The listing builds one solid part. Answer for the finished solid, in the listing's coordinates (mm). Face numbers are marked on the shaded views. A direction names the side the tool comes from. Round coordinates to 2 decimals unless told otherwise and drop trailing zeros. One line per item, written item: value.
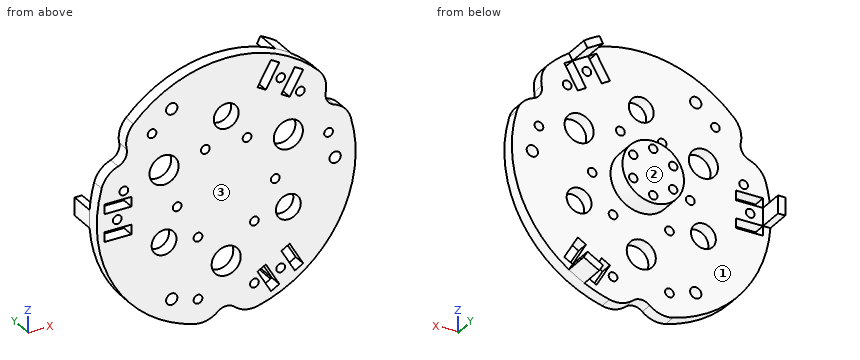
```python
from build123d import *

# Parameters (mm, degrees)
SKETCH1_R                = 50.5
BOSS_EXTRUDE1_DEPTH      = 5
SKETCH3_R                = 12
SKETCH3_R_2              = 1.65
BOSS_EXTRUDE2_DEPTH      = 8
CUT_EXTRUDE6_REACH       = 73.864
SKETCH9_R                = 5.675
SKETCH9_R_2              = 1.7
CIRPATTERN1_COUNT        = 3
SKETCH10_R               = 4.85
CUT_EXTRUDE7_DEPTH       = 72.864455748
SKETCH11_R               = 1.7
CUT_EXTRUDE8_DEPTH       = 72.864455748
CUT_EXTRUDE9_REACH       = 73.864
SKETCH13_R               = 2.2
CIRPATTERN2_COUNT        = 3
CUT_EXTRUDE11_DEPTH      = 72.864455748
BOSS_EXTRUDE3_DEPTH      = 10
CIRPATTERN3_COUNT        = 3
CUT_EXTRUDE12_DEPTH      = 73.114492302
FILLET1_R                = 10
CIRPATTERN4_COUNT        = 3
FILLET1_OF_CIRPATTERN4_R = 10


with BuildPart() as part:
    # Sketch1 → Boss-Extrude1 (new body)
    with BuildSketch(Plane(origin=(0, 0, 0), x_dir=(1, 0, 0), z_dir=(0, 1, 0))):
        with Locations(Location((0, 0, 0), (0, 0, 270))):
            Circle(SKETCH1_R)
    extrude(amount=BOSS_EXTRUDE1_DEPTH)

    # Sketch3 → Boss-Extrude2 (add)
    with BuildSketch(Plane(origin=(0, 5, 0), x_dir=(1, 0, 0), z_dir=(0, 1, 0))):
        with Locations(Location((0, 0, 0), (0, 0, 270))):
            Circle(SKETCH3_R)
        with Locations(Location((0, 9, 0), (0, 0, 270))):
            Circle(SKETCH3_R_2, mode=Mode.SUBTRACT)
        with Locations(Location((7.794228634, 4.5, 0), (0, 0, 270))):
            Circle(SKETCH3_R_2, mode=Mode.SUBTRACT)
        with Locations(Location((7.794228634, -4.5, 0), (0, 0, 270))):
            Circle(SKETCH3_R_2, mode=Mode.SUBTRACT)
        with Locations(Location((0, -9, 0), (0, 0, 270))):
            Circle(SKETCH3_R_2, mode=Mode.SUBTRACT)
        with Locations(Location((-7.794228634, -4.5, 0), (0, 0, 270))):
            Circle(SKETCH3_R_2, mode=Mode.SUBTRACT)
        with Locations(Location((-7.794228634, 4.5, 0), (0, 0, 270))):
            Circle(SKETCH3_R_2, mode=Mode.SUBTRACT)
    extrude(amount=BOSS_EXTRUDE2_DEPTH)

    # Sketch9 → Cut-Extrude6 (cut, up to next)
    with BuildSketch(Plane(origin=(0, 5, 0), x_dir=(1, 0, 0), z_dir=(0, 1, 0)), mode=Mode.PRIVATE) as cut_extrude6_sk1:
        with Locations(Location((0, 28, 0), (0, 0, 270))):
            Circle(SKETCH9_R)
    cut_extrude6_tool1 = extrude(cut_extrude6_sk1.sketch, amount=-CUT_EXTRUDE6_REACH, mode=Mode.PRIVATE) & part.part
    # Sketch9 → Cut-Extrude6 (cut, up to next)
    with BuildSketch(Plane(origin=(0, 5, 0), x_dir=(1, 0, 0), z_dir=(0, 1, 0)), mode=Mode.PRIVATE) as cut_extrude6_sk2:
        with Locations(Location((11, 15.75, 0), (0, 0, 270))):
            Circle(SKETCH9_R_2)
    cut_extrude6_tool2 = extrude(cut_extrude6_sk2.sketch, amount=-CUT_EXTRUDE6_REACH, mode=Mode.PRIVATE) & part.part
    # Sketch9 → Cut-Extrude6 (cut, up to next)
    with BuildSketch(Plane(origin=(0, 5, 0), x_dir=(1, 0, 0), z_dir=(0, 1, 0)), mode=Mode.PRIVATE) as cut_extrude6_sk3:
        with Locations(Location((-11, 15.75, 0), (0, 0, 270))):
            Circle(SKETCH9_R_2)
    cut_extrude6_tool3 = extrude(cut_extrude6_sk3.sketch, amount=-CUT_EXTRUDE6_REACH, mode=Mode.PRIVATE) & part.part
    # Sketch9 → Cut-Extrude6 (cut, up to next)
    with BuildSketch(Plane(origin=(0, 5, 0), x_dir=(1, 0, 0), z_dir=(0, 1, 0)), mode=Mode.PRIVATE) as cut_extrude6_sk4:
        with Locations(Location((11, 39.75, 0), (0, 0, 270))):
            Circle(SKETCH9_R_2)
    cut_extrude6_tool4 = extrude(cut_extrude6_sk4.sketch, amount=-CUT_EXTRUDE6_REACH, mode=Mode.PRIVATE) & part.part
    # Sketch9 → Cut-Extrude6 (cut, up to next)
    with BuildSketch(Plane(origin=(0, 5, 0), x_dir=(1, 0, 0), z_dir=(0, 1, 0)), mode=Mode.PRIVATE) as cut_extrude6_sk5:
        with Locations(Location((-11, 39.75, 0), (0, 0, 270))):
            Circle(SKETCH9_R_2)
    cut_extrude6_tool5 = extrude(cut_extrude6_sk5.sketch, amount=-CUT_EXTRUDE6_REACH, mode=Mode.PRIVATE) & part.part
    cut_extrude6_1 = cut_extrude6_tool1.solids().sort_by_distance((0, 5, -28))[0]
    add(cut_extrude6_1, mode=Mode.SUBTRACT)
    cut_extrude6_2 = cut_extrude6_tool2.solids().sort_by_distance((11, 5, -15.75))[0]
    add(cut_extrude6_2, mode=Mode.SUBTRACT)
    cut_extrude6_3 = cut_extrude6_tool3.solids().sort_by_distance((-11, 5, -15.75))[0]
    add(cut_extrude6_3, mode=Mode.SUBTRACT)
    cut_extrude6_4 = cut_extrude6_tool4.solids().sort_by_distance((11, 5, -39.75))[0]
    add(cut_extrude6_4, mode=Mode.SUBTRACT)
    cut_extrude6_5 = cut_extrude6_tool5.solids().sort_by_distance((-11, 5, -39.75))[0]
    add(cut_extrude6_5, mode=Mode.SUBTRACT)
    cut_extrude6 = cut_extrude6_1 + cut_extrude6_2 + cut_extrude6_3 + cut_extrude6_4 + cut_extrude6_5  # Cut-Extrude6 as one shape, for the pattern or mirror that repeats it

    # CirPattern1: Cut-Extrude6 ×3 about axis
    cirpattern1_axis = Axis((0, 0, 0), (0, 1, 0))
    for i in range(1, CIRPATTERN1_COUNT):
        add(cut_extrude6.rotate(cirpattern1_axis, i * 360 / CIRPATTERN1_COUNT), mode=Mode.SUBTRACT)

    # Sketch10 → Cut-Extrude7 (cut, through all)
    with BuildSketch(Plane(origin=(0, 5, 0), x_dir=(1, 0, 0), z_dir=(0, 1, 0))):
        with Locations(Location((-24.248711306, 14, 0), (0, 0, 270))):
            Circle(SKETCH10_R)
        with Locations(Location((24.248711306, 14, 0), (0, 0, 270))):
            Circle(SKETCH10_R)
        with Locations(Location((0, -28, 0), (0, 0, 270))):
            Circle(SKETCH10_R)
    extrude(amount=-CUT_EXTRUDE7_DEPTH, mode=Mode.SUBTRACT)

    # Sketch11 → Cut-Extrude8 (cut, through all)
    with BuildSketch(Plane(origin=(0, 5, 0), x_dir=(1, 0, 0), z_dir=(0, 1, 0))):
        with Locations(Location((21.25, 36.806079661, 0), (0, 0, 270))):
            Circle(SKETCH11_R)
    cut_extrude8 = extrude(amount=-CUT_EXTRUDE8_DEPTH, mode=Mode.SUBTRACT)

    # Sketch13 → Cut-Extrude9 (cut, up to next)
    with BuildSketch(Plane(origin=(0, 5, 0), x_dir=(1, 0, 0), z_dir=(0, 1, 0)), mode=Mode.PRIVATE) as cut_extrude9_sk1:
        with Locations(Location((-21.25, 36.806079661, 0), (0, 0, 270))):
            Circle(SKETCH13_R)
    cut_extrude9_tool1 = extrude(cut_extrude9_sk1.sketch, amount=-CUT_EXTRUDE9_REACH, mode=Mode.PRIVATE) & part.part
    cut_extrude9 = cut_extrude9_tool1.solids().sort_by_distance((-21.25, 5, -36.80608))[0]
    add(cut_extrude9, mode=Mode.SUBTRACT)

    # CirPattern2: Cut-Extrude8, Cut-Extrude9 ×3 about axis
    cirpattern2_axis = Axis((0, 0, 0), (0, 1, 0))
    add([cut_extrude8.rotate(cirpattern2_axis, i * 360 / CIRPATTERN2_COUNT) for i in range(1, CIRPATTERN2_COUNT)], mode=Mode.SUBTRACT)
    add([cut_extrude9.rotate(cirpattern2_axis, i * 360 / CIRPATTERN2_COUNT) for i in range(1, CIRPATTERN2_COUNT)], mode=Mode.SUBTRACT)

    # Sketch15 → Cut-Extrude11 (cut, through all)
    with BuildSketch(Plane(origin=(0, 5, 0), x_dir=(1, 0, 0), z_dir=(0, 1, 0))):
        Polygon((20.718911087, 42.88620668), (17.471315823, 44.76120668), (12.221315823, 35.66793994), (15.468911087, 33.79293994), align=None)
        Polygon((26.781088913, 39.38620668), (30.028684177, 37.51120668), (24.778684177, 28.41793994), (21.531088913, 30.29293994), align=None)
    cut_extrude11 = extrude(amount=-CUT_EXTRUDE11_DEPTH, mode=Mode.SUBTRACT)

    # Sketch17 → Boss-Extrude3 (add)
    with BuildSketch(Plane(origin=(0, 5, 0), x_dir=(1, 0, 0), z_dir=(0, 1, 0))):
        with BuildLine():
            Line((20.718911087, 42.88620668), (26.781088913, 39.38620668))
            Line((26.781088913, 39.38620668), (28.220372349, 41.879118717))
            ThreePointArc((28.220372349, 41.879118717), (25.25, 43.734282891), (22.158194522, 45.379118717))
            Line((22.158194522, 45.379118717), (20.718911087, 42.88620668))
        make_face()
    boss_extrude3 = extrude(amount=BOSS_EXTRUDE3_DEPTH)

    # CirPattern3: Cut-Extrude11, Boss-Extrude3 ×3 about axis
    cirpattern3_axis = Axis((0, 0, 0), (0, 1, 0))
    add([cut_extrude11.rotate(cirpattern3_axis, i * 360 / CIRPATTERN3_COUNT) for i in range(1, CIRPATTERN3_COUNT)], mode=Mode.SUBTRACT)
    add([boss_extrude3.rotate(cirpattern3_axis, i * 360 / CIRPATTERN3_COUNT) for i in range(1, CIRPATTERN3_COUNT)])

    # Sketch18 → Cut-Extrude12 (cut, through all)
    with BuildSketch(Plane(origin=(0, 5, 0), x_dir=(1, 0, 0), z_dir=(0, 1, 0))):
        with BuildLine():
            ThreePointArc((41.022985472, -29.45105538), (43.734282891, -25.25), (46.016854863, -20.801419868))
            ThreePointArc((46.016854863, -20.801419868), (39.404155872, -22.75), (41.022985472, -29.45105538))
        make_face()
    cut_extrude12 = extrude(amount=-CUT_EXTRUDE12_DEPTH, mode=Mode.SUBTRACT)

    # Fillet1
    fillet1_edges = [part.edges().sort_by_distance(p)[0] for p in [
        (41.022985472, 2.5, 29.45105538),
        (46.016854863, 2.5, 20.801419868),
    ]]
    fillet(fillet1_edges, radius=FILLET1_R)

    # CirPattern4: Cut-Extrude12 ×3 about axis
    cirpattern4_axis = Axis((0, 0, 0), (0, 1, 0))
    for i in range(1, CIRPATTERN4_COUNT):
        add(cut_extrude12.rotate(cirpattern4_axis, i * 360 / CIRPATTERN4_COUNT), mode=Mode.SUBTRACT)

    # Fillet1 of CirPattern4
    fillet1_of_cirpattern4_edges = [part.edges().sort_by_distance(p)[0] for p in [
        (4.993869391, 2.5, -50.252475248),
        (-4.993869391, 2.5, -50.252475248),
        (-46.016854863, 2.5, 20.801419868),
        (-41.022985472, 2.5, 29.45105538),
    ]]
    fillet(fillet1_of_cirpattern4_edges, radius=FILLET1_OF_CIRPATTERN4_R)


solid = part.part
```
1) Each of these flat-tipped pins is pushed along its axis until it touches: pin 1 Ø1.9 at (y, z) = (3, -6.5) entering from -X; pin 2 Ø8 at (x, y) = (32.5, 9.5) entering from -Z; pin 3 Ø5.5 at (x, y) = (-42, 1.5) entering from -Z; pin 4 Ø1.5 at (x, z) = (34, -28.5) entering from +Y. Where does it stop, or does it pass through?
Final values:
pin 1: x = -50.19
pin 2: through
pin 3: z = -31.78
pin 4: y = 5
2) A cutting plane is placed at A-A on y = 8.25. Give the number of separate pieces and of enclosed holes in the cut face, and give its area (3 significant figures).
Final values:
separate pieces: 4
enclosed holes: 6
area: 463 mm2
3) For the marked faces 1, 2 and 3, determine the directions among +Z, -Z, +X, -X, +Y, -Y from which every point of the face is accessible in a straight line to the end or side of a thin tool.
Final values:
face 1: +Y
face 2: +Z, -Z, +X, +Y
face 3: +Z, -Z, +X, -X, -Y
4) Consider L1, parallel to Z at x = -22.5, y = 4; L2, parallel to X at y = 2, z = -15.75; L3, parallel to Z at x = -9, y = 11.25. Determine where each line is inside the solid, lowest interval first.
Final values:
L1: -45.21 to -38.62, -35 to -18.52, -9.48 to 8.6, 19.4 to 35, 38.62 to 45.21
L2: -47.98 to -28.77, -19.73 to -12.7, -9.3 to 9.3, 12.7 to 19.73, 28.77 to 47.98
L3: -7.94 to -5.63, -3.37 to 3.37, 5.63 to 7.94
